Can you work these out from the model? Positions are in its coordinate system, mm. Face numbers are marked on the shaded views. Give positions to 0.01 mm unless a question says otherwise; leave off trailing zeros. Loops run counter-clockwise (first coordinate to the right, second up) from the corner with the lowest first, then second, coordinate; pieces in that order, holes last. Notation, with made-up numbers: (58.25, -6) - (82.25, -6) arc R13 cw to (82.25, 11) - close; hole circle Ø11 at (12, 70). An arc over 180 degrees is marked (long way). Answer as a JSON object with one key per item and string values.
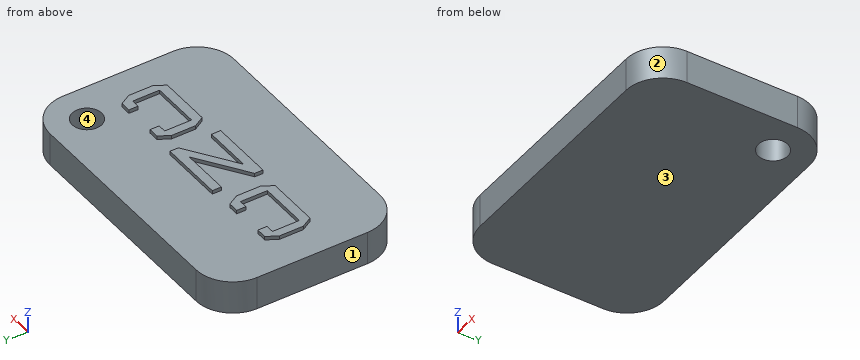
```python
from build123d import *

# Parameters (mm, degrees)
F0_R     = 2
F1_DEPTH = 5
F2_W     = 42.5312
F2_H     = 26.740546
F2_R     = 2
F3_DEPTH = 0.5


with BuildPart() as f1:
    # F0 (on Top) → F1 (new body)
    with BuildSketch(Plane.XY):
        with BuildLine():
            Line((15, 12.5), (-15, 12.5))
            ThreePointArc((-15, 12.5), (-18.535534, 11.035534), (-20, 7.5))
            Line((-20, 7.5), (-20, -7.5))
            ThreePointArc((-20, -7.5), (-18.535534, -11.035534), (-15, -12.5))
            Line((-15, -12.5), (15, -12.5))
            ThreePointArc((15, -12.5), (18.535534, -11.035534), (20, -7.5))
            Line((20, -7.5), (20, 7.5))
            ThreePointArc((20, 7.5), (18.535534, 11.035534), (15, 12.5))
        make_face()
        with Locations((15, 7.5)):
            Circle(F0_R, mode=Mode.SUBTRACT)
    extrude(amount=F1_DEPTH)

    # F2 (on face) → F3 (cut)
    with BuildSketch(Plane.XY.offset(5)):
        Rectangle(F2_W, F2_H)
        with BuildLine():
            Line((-15, 12.5), (15, 12.5))
            ThreePointArc((15, 12.5), (18.535534, 11.035534), (20, 7.5))
            Line((20, 7.5), (20, -7.5))
            ThreePointArc((20, -7.5), (18.535534, -11.035534), (15, -12.5))
            Line((15, -12.5), (-15, -12.5))
            ThreePointArc((-15, -12.5), (-18.535534, -11.035534), (-20, -7.5))
            Line((-20, -7.5), (-20, 7.5))
            ThreePointArc((-20, 7.5), (-18.535534, 11.035534), (-15, 12.5))
        make_face(mode=Mode.SUBTRACT)
        with Locations((15, 7.5)):
            Circle(F2_R)
        with BuildLine():
            ThreePointArc((20, 7.5), (18.535534, 11.035534), (15, 12.5))
            Line((15, 12.5), (-15, 12.5))
            ThreePointArc((-15, 12.5), (-18.535534, 11.035534), (-20, 7.5))
            Line((-20, 7.5), (-20, -7.5))
            ThreePointArc((-20, -7.5), (-18.535534, -11.035534), (-15, -12.5))
            Line((-15, -12.5), (15, -12.5))
            ThreePointArc((15, -12.5), (18.535534, -11.035534), (20, -7.5))
            Line((20, -7.5), (20, 7.5))
        make_face()
        Polygon((-7.840759, 1.722246), (-8.956835, 1.722246), (-8.956835, 2.966643), (-7.551199, 2.966643), (-6.720365, 1.523822), (-6.720365, -1.746251), (-7.551199, -3.189047), (-14.715777, -3.189047), (-15.550929, -1.746251), (-15.550929, 1.523822), (-14.715777, 2.966643), (-13.310141, 2.966643), (-13.310141, 1.722246), (-14.430535, 1.722246), (-14.430535, -1.944701), (-7.840759, -1.944701), align=None, mode=Mode.SUBTRACT)
        Polygon((-2.267872, -2.351202), (-2.267872, -2.376044), (4.309483, -2.376044), (4.309483, -3.62039), (-4.396925, -3.62039), (-4.396925, -2.491791), (2.18457, 2.010257), (2.18457, 2.035098), (-4.396925, 2.035098), (-4.396925, 3.279444), (4.309483, 3.279444), (4.309483, 2.146706), align=None, mode=Mode.SUBTRACT)
        Polygon((14.343017, 1.722246), (13.226788, 1.722246), (13.226788, 2.966643), (14.632399, 2.966643), (15.463335, 1.523822), (15.463335, -1.746251), (14.632399, -3.189047), (7.467973, -3.189047), (6.632872, -1.746251), (6.632872, 1.523822), (7.467973, 2.966643), (8.873559, 2.966643), (8.873559, 1.722246), (7.753241, 1.722246), (7.753241, -1.944701), (14.343017, -1.944701), align=None, mode=Mode.SUBTRACT)
        with Locations((15, 7.5)):
            Circle(F2_R, mode=Mode.SUBTRACT)
    extrude(amount=-F3_DEPTH, mode=Mode.SUBTRACT)


solid = f1.part
```
1) Imagine slicing it at C-C on y = 4.25. Write out the boundary of the cut face in (x, z), and give its area (3 significant figures).
Check sheet entries:
{"outline": "(-20, 0) - (20, 0) - (20, 4.5) - (-20, 4.5) - close", "area": "180 mm2"}
2) I need wall thicknesses on L1, parallel to Y at x = 15, z = 2.15; L2, parallel to Z at x = 5, y = -0.5; L3, parallel to X at y = 8.5, z = 0.6. Which ranges of each line are inside material? Lowest first, please.
Check sheet entries:
{"L1": "-12.5 to 5.5, 9.5 to 12.5", "L2": "0 to 4.5", "L3": "-19.9 to 13.27, 16.73 to 19.9"}
3) If we mould it in two halves opening along X, with no side actions, what happens to the marked faces 1, 2, 3 and 4? For each: released by +X, released by -X, zero draft, split by the parting line, or undercut.
Check sheet entries:
{"face 1": "released by -X", "face 2": "released by +X", "face 3": "zero draft", "face 4": "undercut"}
4) Imagine slicing it at B-B on x = -8.5. Write out the boundary of the cut face in (y, z).
Check sheet entries:
{"outline": "(-12.5, 0) - (12.5, 0) - (12.5, 4.5) - (2.97, 4.5) - (2.97, 5) - (1.72, 5) - (1.72, 4.5) - (-1.94, 4.5) - (-1.94, 5) - (-3.19, 5) - (-3.19, 4.5) - (-12.5, 4.5) - close"}
5) I'm going to push flat-ended pins straight in: P1, Ø1.5, axis at y = 10, z = 2, coming from the -X side; P2, Ø0.6, axis at x = -11, z = 5, coming from the +Y side; P3, Ø10, axis at x = 6, y = -5, coming from the +Z side; P4, Ø0.6, axis at y = -0.5, z = 5, coming from the -X side. Where does each tip first touch, or does it pass through?
Check sheet entries:
{"P1": "x = -19.68", "P2": "y = -1.94", "P3": "z = 5", "P4": "x = -15.55"}
6) Imagine slicing it at D-D on y = 10.75. Write out the boundary of the cut face in (x, z).
Check sheet entries:
{"outline": "(-18.8, 0) - (18.8, 0) - (18.8, 4.5) - (-18.8, 4.5) - close"}
7) Imagine slicing it at A-A on z = 1.15. Write out the boundary of the cut face in (x, y).
Check sheet entries:
{"outline": "(-20, -7.5) arc R5 ccw to (-15, -12.5) - (15, -12.5) arc R5 ccw to (20, -7.5) - (20, 7.5) arc R5 ccw to (15, 12.5) - (-15, 12.5) arc R5 ccw to (-20, 7.5) - close; hole circle Ø4 at (15, 7.5)"}
